Here's how the part is built. I have some questions about the finished solid (model axes, mm). A direction names the side the tool comes from. Round coordinates to 2 decimals unless told otherwise and drop trailing zeros. Loops run counter-clockwise (first coordinate to the right, second up) from the corner with the lowest first, then second, coordinate; pieces in that order, holes last. Notation, with made-up numbers: M -40,73.25 L -8,73.25 A36 ccw -8,110.25 Z; hole C 37.25,14.25 d2. An arc over 180 degrees is marked long. Write each question's results on one line, items separated by ' | '. Start each with the question number.
```python
from build123d import *

# Parameters (mm, degrees)
SKETCH1_R               = 30
BOSS_EXTRUDE1_DEPTH     = 10
SKETCH2_R               = 25
CUT_EXTRUDE1_DEPTH      = 2
SKETCH3_R               = 6.625
CUT_EXTRUDE2_DEPTH      = 5
SKETCH4_R               = 3.75
CUT_EXTRUDE4_DEPTH      = 8
CUT_EXTRUDE4_DEPTH_BACK = 4


with BuildPart() as part:
    # Sketch1 → Boss-Extrude1 (new body)
    with BuildSketch(Plane(origin=(0, 0, 0), x_dir=(1, 0, 0), z_dir=(0, 1, 0))):
        Circle(SKETCH1_R)
    extrude(amount=BOSS_EXTRUDE1_DEPTH)

    # Sketch2 → Cut-Extrude1 (cut)
    with BuildSketch(Plane(origin=(0, 10, 0), x_dir=(1, 0, 0), z_dir=(0, 1, 0))):
        Circle(SKETCH2_R)
    extrude(amount=-CUT_EXTRUDE1_DEPTH, mode=Mode.SUBTRACT)

    # Sketch3 → Cut-Extrude2 (cut)
    with BuildSketch(Plane(origin=(0, 8, 0), x_dir=(1, 0, 0), z_dir=(0, 1, 0))):
        Circle(SKETCH3_R)
    extrude(amount=-CUT_EXTRUDE2_DEPTH, mode=Mode.SUBTRACT)

    # Sketch4 → Cut-Extrude4 (cut, two sides)
    with BuildSketch(Plane(origin=(0, 3, 0), x_dir=(1, 0, 0), z_dir=(0, 1, 0))) as cut_extrude4_sk:
        Circle(SKETCH4_R)
    extrude(amount=CUT_EXTRUDE4_DEPTH, mode=Mode.SUBTRACT)
    extrude(cut_extrude4_sk.sketch, amount=-CUT_EXTRUDE4_DEPTH_BACK, mode=Mode.SUBTRACT)


solid = part.part
```
Item 1: If we section it at D-D on x = 12: Please give me the cut outline in (y, z).
Item 2: I'm going to push flat-ended pins straight in: pin 1 (5 mm diameter, centred on x = -2, y = 4, fed in from +Z); pin 2 (1.5 mm diameter, centred on x = 5.5, z = 5, fed in from -Y); pin 3 (3 mm diameter, centred on x = -2.5, z = 22.5, fed in from +Y); pin 4 (2 mm diameter, centred on y = 4.5, z = -5.5, fed in from +X). Where does each tip first touch, or does it pass through?
Item 3: I need wall thicknesses on L1, parallel to X at y = 9.4, z = 0; L2, parallel to X at y = 4.1, z = 0 (3 decimals). Which ranges of each line are inside material? Lowest first, please.
Item 4: If we section it at C-C on y = 1: Please give me the cut outline in (x, z).
Item 5: If we mould it in two halves opening along Z, with no side actions, what happens to faces 3 (the face through (-7, 10, -25)), 4 (the face through (-29.97, 4.93, -1.32)), 5 (the face through (3, 3, 3))? For each: released by +Z, released by -Z, zero draft, split by the parting line, or undercut.
Item 6: If we section it at A-A on x = 0: Please give me the cut outline in (y, z) (3 decimals), and give its area (3 significant figures).
Item 7: Which directions (+Z, -Z, +X, -X, +Y, -Y) give clear straight access to the entire face, cutting with the end or side of a thin tool? Please do faces 1 (the face through (6, 0, 0)), 2 (the face through (3.562, 5.535, -5.586)).
Item 8: If we section it at B-B on z = 0: Please give me the cut outline in (x, y) (3 decimals), and give its area (3 significant figures).
Numbers:
1) outline: M 0,-27.5 L 10,-27.5 L 10,-21.93 L 8,-21.93 L 8,21.93 L 10,21.93 L 10,27.5 L 0,27.5 Z
2) pin 1: z = 30 | pin 2: y = 0 | pin 3: y = 8 | pin 4: x = 29.66
3) L1: -30 to -25, 25 to 30 | L2: -30 to -6.625, 6.625 to 30
4) outline: C 0,0 d60; hole C 0,0 d7.5
5) face 3: zero draft | face 4: split by the parting line | face 5: undercut
6) outline: M 0,-30 L 10,-30 L 10,-25 L 8,-25 L 8,-6.625 L 3,-6.625 L 3,-3.75 L 0,-3.75 Z; M 0,3.75 L 3,3.75 L 3,6.625 L 8,6.625 L 8,25 L 10,25 L 10,30 L 0,30 Z | area: 411 mm²
7) face 1: +Z, -Z, +X, -X, -Y | face 2: +Y
8) outline: M -30,0 L -3.75,0 L -3.75,3 L -6.625,3 L -6.625,8 L -25,8 L -25,10 L -30,10 Z; M 3.75,0 L 30,0 L 30,10 L 25,10 L 25,8 L 6.625,8 L 6.625,3 L 3.75,3 Z | area: 411 mm²
